Geometry: see drawing. Coordinates: mm, zero at the bounding-box minimum. Give positions to 0.01 mm unless a question says otherwise; leave off trailing zeros. Write each loop counter-clockwise with the first axis right and the second up, starting at its lowest first coordinate (ties: lowest second). Pieces come first, ordered by that corner, then holes. Notation, with made-up numbers: (51, 30) -> (64, 30) arc R28 cw to (64, 66) -> close; hole circle Ø9 at (49.5, 28). An arc over 180 degrees is marked (long way). Answer as a JSON object with one key per item and string values. Group by question number.
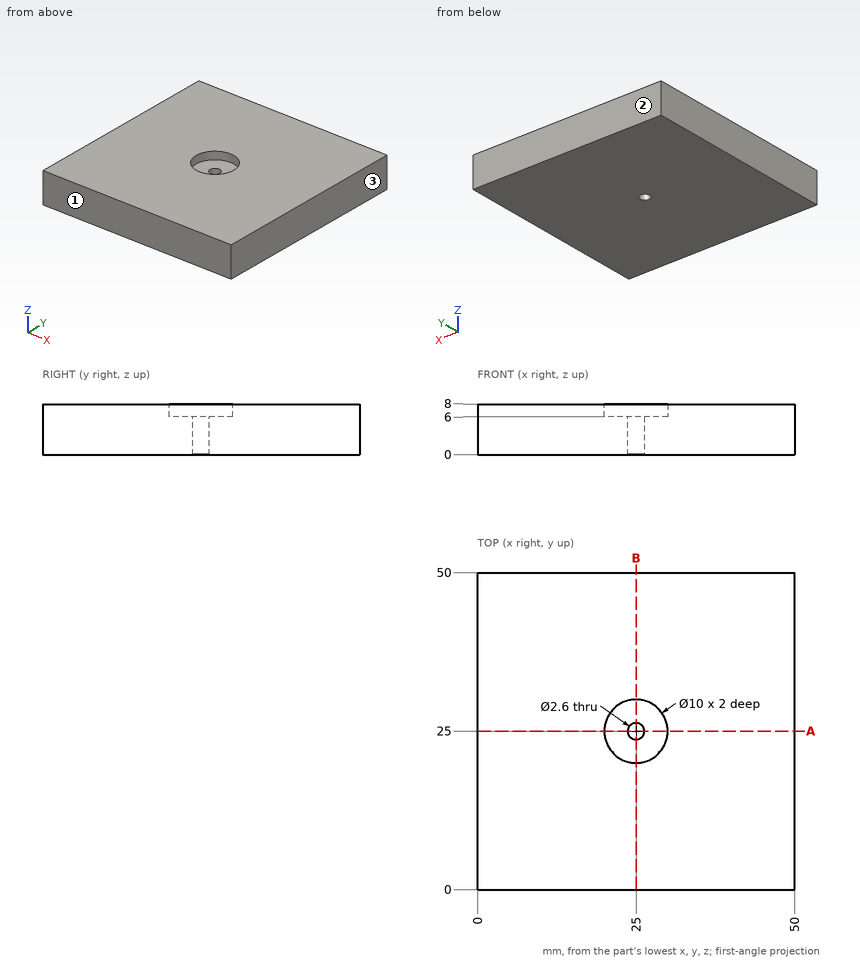
1. Line query: line 1 (Y direction, x = 25, z = 6.9); line 2 (Y direction, x = 25, z = 2.5); line 3 (Z direction, x = 28, y = 28). Output: solid intervals per line, ascending.
2. Section A-A (y = 25). Return the cut outline in (x, z).
3. Mould query, pull axis Y, two halves, no side actions, for the marked faces 1, 2 and 3. Classes: pulls with the +Y half, pulls with the -Y half, needs draft (parallel to the pull), parting line crosses it, or undercut.
4. Contact query for flat-ended pins moving along their axis: pin 1 Ø2.5 at (x, y) = (25, 25) entering from -Z; pin 2 Ø9 at (x, y) = (25, 25) entering from +Z. Output: stop coordinate, or through.
Working result:
{
 "1": {"line 1": "y = 0 to 20, 30 to 50", "line 2": "y = 0 to 23.7, 26.3 to 50", "line 3": "z = 0 to 6"},
 "2": {"outline": "(0, 0) -> (23.7, 0) -> (23.7, 6) -> (20, 6) -> (20, 8) -> (0, 8) -> close; (26.3, 0) -> (50, 0) -> (50, 8) -> (30, 8) -> (30, 6) -> (26.3, 6) -> close"},
 "3": {"face 1": "pulls with the -Y half", "face 2": "pulls with the +Y half", "face 3": "needs draft"},
 "4": {"pin 1": "passes through", "pin 2": "stops at z = 6"}
}
